The model under review builds one solid part; all positions refer to its coordinate system, in mm. Face numbers are marked on the shaded views. A direction names the side the tool comes from. Round coordinates to 2 decimals unless told otherwise and drop trailing zeros. Order: outer loops, then holes, each group sorted by start corner. A loop starts at its lowest first (then second) coordinate and runs counter-clockwise, first axis right, second up.
```python
from build123d import *

# Parameters (mm, degrees)
F1_DEPTH       = 76.2
F3_DEPTH       = 27.94
F4_R           = 10.16
F5_DEPTH       = 76.201
F7_DEPTH       = 10.16
F8_D           = 15.24
F8_CBORE_D     = 40.64
F8_CBORE_DEPTH = 10.16
F9_R           = 10.16


with BuildPart() as f1:
    # F0 (on Front) → F1 (new body)
    with BuildSketch(Plane.XZ):
        Polygon((0, 35.56), (0, 0), (111.76, 0), (147.32, 35.56), (147.32, 71.12), (111.76, 71.12), (76.2, 35.56), align=None)
    extrude(amount=-F1_DEPTH)

    # F2 (on face) → F3 (cut)
    with BuildSketch(Plane.XY.offset(71.12)):
        with BuildLine():
            ThreePointArc((125.73, 15.24), (129.54, 11.43), (133.35, 15.24))
            Line((133.35, 15.24), (133.35, 60.96))
            ThreePointArc((133.35, 60.96), (129.54, 64.77), (125.73, 60.96))
            Line((125.73, 60.96), (125.73, 15.24))
        make_face()
    extrude(amount=-F3_DEPTH, mode=Mode.SUBTRACT)

    # F4 (on face) → F5 (cut, through all)
    with BuildSketch(Plane.XZ):
        with Locations((93.98, 20.32)):
            Circle(F4_R)
    extrude(amount=-F5_DEPTH, mode=Mode.SUBTRACT)

    # F6 (on face) → F7 (cut)
    with BuildSketch(Plane.XY.offset(35.56)):
        with BuildLine():
            ThreePointArc((18.425245, 33.02), (17.78, 38.1), (18.425245, 43.18))
            Line((18.425245, 43.18), (0, 43.18))
            Line((0, 43.18), (0, 33.02))
            Line((0, 33.02), (18.425245, 33.02))
        make_face()
        with BuildLine():
            ThreePointArc((57.774755, 43.18), (58.258043, 40.660407), (58.42, 38.1))
            ThreePointArc((58.42, 38.1), (58.258043, 35.539593), (57.774755, 33.02))
            Line((57.774755, 33.02), (76.2, 33.02))
            Line((76.2, 33.02), (76.2, 43.18))
            Line((76.2, 43.18), (57.774755, 43.18))
        make_face()
    extrude(amount=-F7_DEPTH, mode=Mode.SUBTRACT)

    # F8 (through all)
    with Locations(Plane.XY.offset(35.56)):
        with Locations((38.1, 38.1)):
            CounterBoreHole(F8_D / 2, F8_CBORE_D / 2, F8_CBORE_DEPTH)

    # F9
    f9_edges = [f1.edges().sort_by_distance(p)[0] for p in [
        (0, 0, 17.78),
        (0, 76.2, 17.78),
    ]]
    fillet(f9_edges, radius=F9_R)


solid = f1.part
```
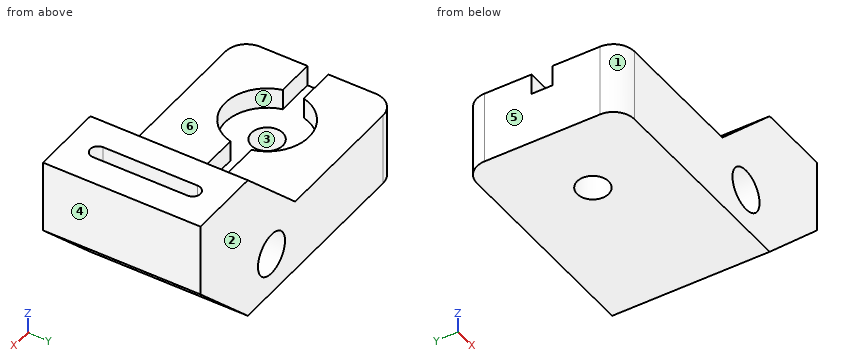
(1) Consider section A-A (z = 20.32). Write out the cut boundary in (x, y).
Data:
outline: (0, 10.16) arc R10.16 ccw to (10.16, 0) - (83.82, 0) - (83.82, 76.2) - (10.16, 76.2) arc R10.16 ccw to (0, 66.04) - close; (104.14, 0) - (132.08, 0) - (132.08, 76.2) - (104.14, 76.2) - close; hole circle Ø15.24 at (38.1, 38.1)
(2) For the marked faces 5, 6 and 7, list the 3-axis set-ups (+Z, -Z, +X, -X, +Y, -Y) from which the entire face can be reached by the end or side of a thin tool; tool diameter is ignored.
Data:
face 5: +Z, -Z, -X, +Y, -Y
face 6: +Z, -X, +Y, -Y
face 7: +Z
(3) Consider section B-B (x = 38.1). Write out the cut boundary in (y, z).
Data:
outline: (0, 0) - (30.48, 0) - (30.48, 25.4) - (17.78, 25.4) - (17.78, 35.56) - (0, 35.56) - close; (45.72, 0) - (76.2, 0) - (76.2, 35.56) - (58.42, 35.56) - (58.42, 25.4) - (45.72, 25.4) - close
(4) Consider section D-D (z = 49). Write out the cut boundary in (x, y), and give its area (3 significant figures).
Data:
outline: (89.64, 0) - (147.32, 0) - (147.32, 76.2) - (89.64, 76.2) - close; hole (125.73, 15.24) arc R3.81 ccw to (133.35, 15.24) - (133.35, 60.96) arc R3.81 ccw to (125.73, 60.96) - close
area: 4,000 mm2
(5) Draft analysis for pull direction Y (two halves, no side actions). For the marked faces 1, 2, 3 and 4, state which applies: pulls with the +Y half, pulls with the -Y half, needs draft (parallel to the pull), parting line crosses it, or undercut.
Data:
face 1: pulls with the -Y half
face 2: pulls with the +Y half
face 3: undercut
face 4: needs draft
(6) Insertion check: pin 1 (4 mm diameter, centred on x = 128.5, y = 33.5, fed in from +Z); pin 2 (16.5 mm diameter, centred on x = 24, y = 13.5, fed in from +Z); pin 3 (8.5 mm diameter, centred on y = 37.5, z = 62, fed in from -X). Each pin has a flat end and moves straight along its axis. Give the tip position at first contact, or say it passes through.
Data:
pin 1: stops at z = 43.18
pin 2: stops at z = 35.56
pin 3: stops at x = 98.39
(7) Consider section C-C (x = 129.54). Write out the cut boundary in (y, z).
Data:
outline: (0, 17.78) - (76.2, 17.78) - (76.2, 71.12) - (64.77, 71.12) - (64.77, 43.18) - (11.43, 43.18) - (11.43, 71.12) - (0, 71.12) - close
(8) To check wall thickness, follow probe 1 along Y at (x, z) = (38.1, 15.5); probe 2 along X at (y, z) = (47, 26); probe 3 along X at (y, z) = (26, 25.5). State the ranges of each line that lie inside material, in increasing order.
Data:
probe 1: y = 0 to 30.48, 45.72 to 76.2
probe 2: x = 0 to 19.83, 56.37 to 85.56, 102.4 to 137.76
probe 3: x = 0 to 21.78, 54.42 to 85.24, 102.72 to 137.26
